For this review, take the finished solid that the model builds, in its own axes (mm). Give positions to 0.01 mm unless a question says otherwise; leave off trailing zeros. Write each loop counter-clockwise with the first axis right and the second up, starting at its lowest first coordinate (ties: lowest second). Pieces come first, ordered by that corner, then holes.
1) Wall thickness on line 1 along X through (y, z) = (-4, -3.5); line 2 along Y through (x, z) = (-2, 4.75); line 3 along X through (y, z) = (0.5, -2.5): over which ranges is each line inside the solid? List them lowest first.
2) We need section A-A on z = -0.5. Give the boundary of the cut face in (x, y), and give its area (3 significant figures).
3) For P1, Ø1.2, axis at x = 22.5, z = 3.5, coming from the -Y side; P2, Ø2, axis at x = 19, z = -3, coming from the -Y side; P3, Ø1.5, axis at y = -9.5, z = 1.5, coming from the +X side, all flat-tipped, find the tip position at first contact; note any pin that passes through.
4) We need section C-C on y = -12.25. Give the boundary of the cut face in (x, z), and give its area (3 significant figures).
5) We need section D-D on z = 3. Give the boundary of the cut face in (x, y), and give its area (3 significant figures).
6) We need section B-B on x = 11.5. Give the boundary of the cut face in (y, z).
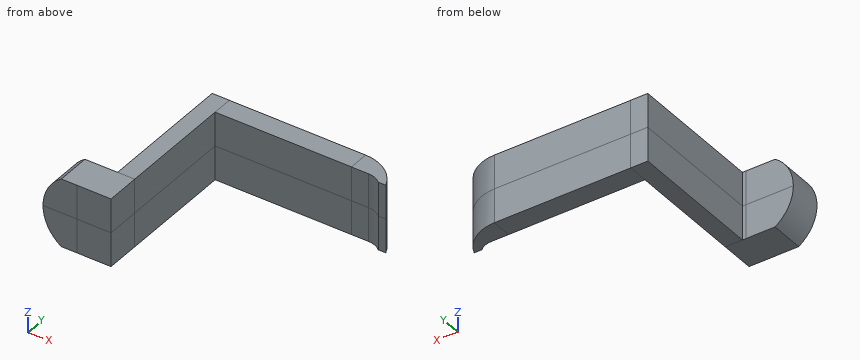
Autodesk Inventor part; units mm, degrees
ref_plane "YZ Plane" through (0, 0, 0) normal (1, 0, 0) x (0, 1, 0)
ref_plane "XZ Plane" through (0, 0, 0) normal (0, 1, 0) x (-1, 0, 0)
ref_plane "XY Plane" through (0, 0, 0) normal (0, 0, 1) x (1, 0, 0)
sketch "Sketch2" plane through (0, 0, 0) normal (0, 0, 1) x (1, 0, 0)
  line L0 (-17.5, -21) -> (-7.5, -21)
  line L1 (-91.1, -16) -> (-5.5, -16)
  line L2 (-5.5, -16) -> (-5.5, 28.3)
  line L3 (-12.5, -21) -> (-12.5, -16)
  line L4 (-12.5, -21) -> (-2.5, -21)
  line L5 (-2.5, -21) -> (-2.5, -15.999)
  line L6 (-2.5, -15.999) -> (-12.5, -15.999)
  line L7 (-12.5, -15.999) -> (-12.5, -21)
  line L8 (-2.5, -15.999) -> (-5.0122, -15.999)
  line L9 (-5.0122, -15.999) -> (-5.0122, 4.001)
  line L10 (-5.0122, 4.001) -> (-2.5, 4.001)
  line L11 (-2.5, 4.001) -> (-2.5, -15.999)
  line L12 (-2.5, 4.001) -> (17.5, 4.001)
  line L13 (17.5, 4.001) -> (17.5, 1.001)
  line L14 (17.5, 1.001) -> (-2.5, 1.001)
  line L15 (-2.5, 1.001) -> (-2.5, 4.001)
  arc A0 (23.0689, 0.2342) -> (17.5, 4.001) centre (17.5, -1.999) ccw
  arc A1 (21.9703, 0.2342) -> (20.0013, 1.001) centre (20.0013, -1.9105) ccw
  line L16 (20.0013, 1.001) -> (17.5, 1.001)
  line L17 (23.0689, 0.2342) -> (21.9703, 0.2342)
  point P0 (0, 0)
  point P1 (-5.5, -15.999)
  dimension "d0" = 10
  dimension "d1" = 20
  dimension "d2" = 20
  dimension "d3" = 3
  dimension "d9" = 6
extrude "Extrusion1" add sketch "Sketch2" against normal mid plane 10
sketch "Sketch3" plane through (-12.5, -21, -5) normal (0, -1, 0) x (1, 0, 0)
  line L0 (5, 0) -> (5, -5)
  line L1 (0, 0) -> (7.4878, 0)
  arc A0 (2.7054, 10) -> (2.7054, 0) centre (6.0221, 5) ccw
  line L2 (2.7054, 0) -> (-2.2946, 0)
  line L3 (0, 0) -> (0, 10)
  line L4 (-2.2946, 10) -> (2.7054, 10)
  line L5 (-2.2946, 0) -> (-2.2946, 10)
  point P0 (12.5, 5)
  point P1 (2.7054, 0)
  dimension "d6" = 6
extrude "Extrusion2" cut sketch "Sketch3" against normal blind 10 contours L3 L4 A0 L1
properties part number "ЛЦМК000002.00.00.00.00.07"
Results list:
1. line 1: x = -5.01 to -2.5
1. line 2: y = 1 to 4
1. line 3: x = -5.01 to -2.5, 21.63 to 22.95
2. outline: (-12.46, -21) - (-2.5, -21) - (-2.5, 1) - (20, 1) arc R2.91 cw to (21.97, 0.23) - (23.07, 0.23) arc R6 ccw to (17.5, 4) - (-5.01, 4) - (-5.01, -16) - (-5.5, -16) - (-12.46, -16) - close
2. area: 172 mm2
3. P1: stops at y = 0.23
3. P2: stops at y = 1
3. P3: stops at x = -2.5
4. outline: (-5.01, -5) - (-2.5, -5) - (-2.5, 5) - (-5.01, 5) - close
4. area: 25.1 mm2
5. outline: (-11.67, -21) - (-2.5, -21) - (-2.5, 1) - (20, 1) arc R2.91 cw to (21.97, 0.23) - (23.07, 0.23) arc R6 ccw to (17.5, 4) - (-5.01, 4) - (-5.01, -16) - (-5.5, -16) - (-11.67, -16) - close
5. area: 168 mm2
6. outline: (1, -5) - (4, -5) - (4, 5) - (1, 5) - close
